The drawing under review shows one solid part. Ordinate dimensions are in mm from its lowest x, y, z. A direction names the side the tool comes from. Round coordinates to 2 decimals unless told otherwise and drop trailing zeros. Write each loop counter-clockwise with the first axis right and the second up, starting at its lowest first coordinate (ties: lowest second). Pieces come first, ordered by that corner, then holes. Notation, with made-up numbers: (14.25, -4.5) -> (53.25, -4.5) arc R23 cw to (53.25, 31.5) -> close; hole circle Ø6 at (68.5, 44.5). An arc over 180 degrees is marked (long way). Answer in a Markdown table with one row per item. Add a question column.
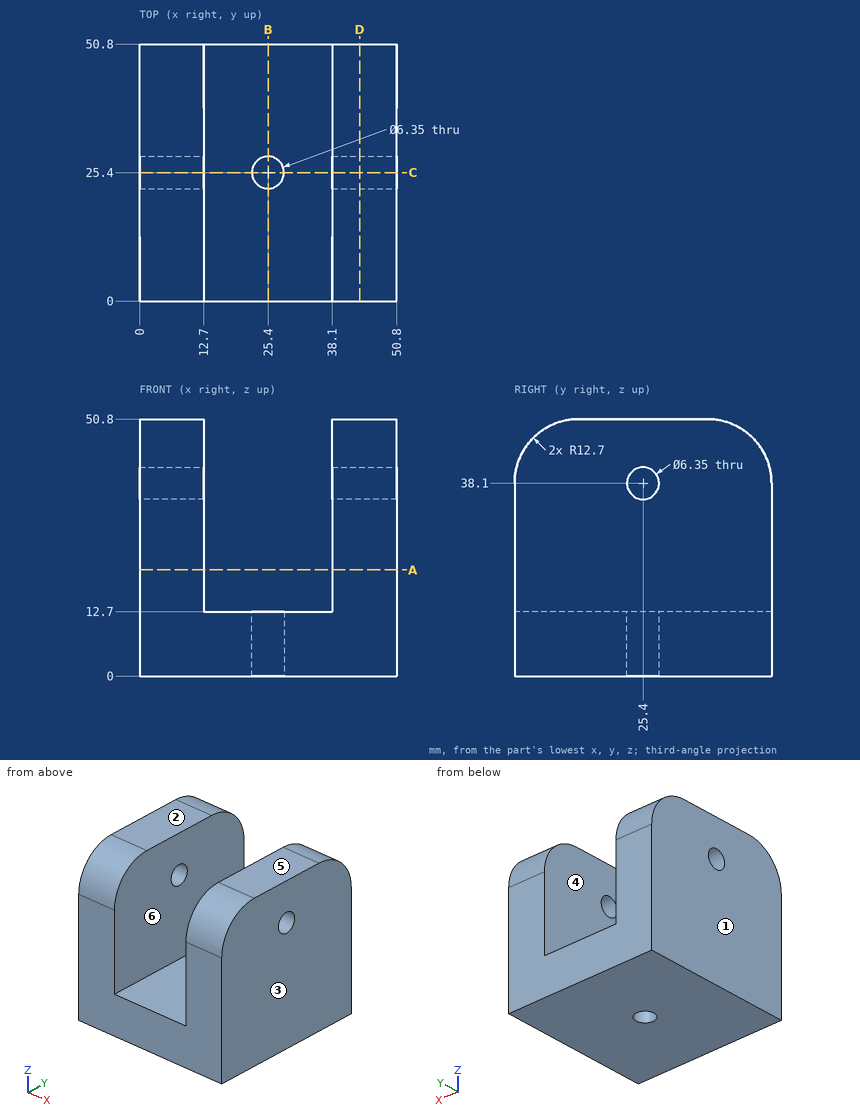
1. Insertion check: pin 1 Ø6 at (x, z) = (34.5, 38) entering from -Y; pin 2 Ø10 at (x, y) = (25.4, 25.4) entering from +Z; pin 3 Ø1 at (x, y) = (12.5, 7.5) entering from +Z. Each pin has a flat end and moves straight along its axis. Give the tip position at first contact, or say it passes through.
2. Add section C-C on y = 25.4. Write out the cut boundary in (x, z) (3 decimals), plus the area to 3 significant figures.
3. For L1, parallel to X at y = 41, z = 22; L2, parallel to Y at x = 5.5, z = 38.1 (3 decimals); L3, parallel to Z at x = 24.5, y = 17.5, list the stretches that pass through material, from the lowest coordinate up.
4. Tool access review of the marked faces 5 and 6: name each direction out of +Z, -Z, +X, -X, +Y, -Y from which nothing blocks a thin tool from reaching the whole face with its end or side.
5. Add section D-D on x = 43.5. Write out the cut boundary in (y, z) (3 decimals).
6. Add section B-B on x = 25.4. Write out the cut boundary in (y, z) (3 decimals).
7. Mouldability with a two-part tool opening along X and no side actions: class the marked faces 1, 2, 3 and 4 as pulls with the +X half, pulls with the -X half, needs draft (parallel to the pull), parting line crosses it, or undercut.
8. Add section A-A on z = 21. Write out the cut boundary in (x, y).
Filled in:
| question | item | result |
|---|---|---|
| 1 | pin 1 | through |
| 1 | pin 2 | z = 12.7 |
| 1 | pin 3 | z = 49.9 |
| 2 | outline | (0, 0) -> (22.225, 0) -> (22.225, 12.7) -> (12.7, 12.7) -> (12.7, 34.925) -> (0, 34.925) -> close; (0, 41.275) -> (12.7, 41.275) -> (12.7, 50.8) -> (0, 50.8) -> close; (28.575, 0) -> (50.8, 0) -> (50.8, 34.925) -> (38.1, 34.925) -> (38.1, 12.7) -> (28.575, 12.7) -> close; (38.1, 41.275) -> (50.8, 41.275) -> (50.8, 50.8) -> (38.1, 50.8) -> close |
| 2 | area | 1,370 mm² |
| 3 | L1 | 0 to 12.7, 38.1 to 50.8 |
| 3 | L2 | 0 to 22.225, 28.575 to 50.8 |
| 3 | L3 | 0 to 12.7 |
| 4 | face 5 | +Z, +X, -X, +Y, -Y |
| 4 | face 6 | +Z, +Y, -Y |
| 5 | outline | (0, 0) -> (50.8, 0) -> (50.8, 38.1) arc R12.7 ccw to (38.1, 50.8) -> (12.7, 50.8) arc R12.7 ccw to (0, 38.1) -> close; hole circle Ø6.35 at (25.4, 38.1) |
| 6 | outline | (0, 0) -> (22.225, 0) -> (22.225, 12.7) -> (0, 12.7) -> close; (28.575, 0) -> (50.8, 0) -> (50.8, 12.7) -> (28.575, 12.7) -> close |
| 7 | face 1 | pulls with the -X half |
| 7 | face 2 | needs draft |
| 7 | face 3 | pulls with the +X half |
| 7 | face 4 | undercut |
| 8 | outline | (0, 0) -> (12.7, 0) -> (12.7, 50.8) -> (0, 50.8) -> close; (38.1, 0) -> (50.8, 0) -> (50.8, 50.8) -> (38.1, 50.8) -> close |
